Model file for the job. Use its own axes, mm. Face numbers are marked on the shaded views. A direction names the side the tool comes from. Coordinates: 2 decimals unless noted, no trailing zeros. Write each loop counter-clockwise with the first axis right and the second up, starting at its lowest first coordinate (ties: lowest second). Pieces come first, ordered by that corner, then holes. Notation, with made-up numbers: M 74.25,42 L 107.25,42 A32 cw 107.25,81 Z; hole C 25,-1.5 d5. An arc over 180 degrees is marked long. Put each result on its own line as item: value. Start each with the question number.
Q1. Cut at C-C (z = 25.25). Write the cut outline in (x, y).
Q2. Cut at D-D (z = 10.25). Write the cut outline in (x, y).
Q3. Cut at B-B (y = 6.2). Write the cut outline in (x, z).
Q4. Cut at A-A (z = 15). Write the cut outline in (x, y), then the cut area to 3 significant figures.
Q5. Drill centre lines: line 1 along X through (y, z) = (8.5, 21.5); line 2 along Z through (x, y) = (5.15, 6.2); line 3 along X through (y, z) = (2, 1.75). Where is each one in solid material? Low to high.
Q6. Drop flat-ended pins along their axis: pin 1 (3 mm diameter, centred on y = 7.5, z = 16.5, fed in from -X); pin 2 (1.5 mm diameter, centred on x = 2.5, y = 5.5, fed in from +Z); pin 3 (4 mm diameter, centred on x = -29, z = 16.5, fed in from +Y). Give the stop position or say it passes through.
Q7. Pull direction X, two halves, no side cores. Call the marked faces 1, 2 and 3: pulls with the +X half, pulls with the -X half, needs draft (parallel to the pull), parting line crosses it, or undercut.
Q8. Which spindle directions (+Z, -Z, +X, -X, +Y, -Y) get a long thin tool onto all of the face, cutting with end or side? Do the marked faces 4, 5 and 6. Say none if no direction does.
```python
from build123d import *

# Parameters (mm, degrees)
F3_DEPTH = 30
F4_R     = 2.2
F5_DEPTH = 6
F6_W     = 3
F6_H     = 8
F7_DEPTH = 19


with BuildPart() as f3:
    # F2 (on Top) → F3 (new body)
    with BuildSketch(Plane.XY):
        Polygon((0, 13), (0, 0), (6, 0), (6, 19), (-26, 19), (-26, -11), (-34, -11), (-34, -31), (-31, -31), (-31, -14), (-20, -14), (-20, 13), align=None)
    extrude(amount=F3_DEPTH)

    # F4 (on face) → F5 (cut)
    with BuildSketch(Plane(origin=(0, 0, 0), x_dir=(0, -1, 0), z_dir=(-1, 0, 0))):
        with Locations((-6.2, 15)):
            Circle(F4_R)
    extrude(amount=-F5_DEPTH, mode=Mode.SUBTRACT)

    # F6 (on face) → F7 (cut)
    with BuildSketch(Plane.XY.offset(30)):
        with Locations((3, 6.3)):
            Rectangle(F6_W, F6_H)
    extrude(amount=-F7_DEPTH, mode=Mode.SUBTRACT)


solid = f3.part
```
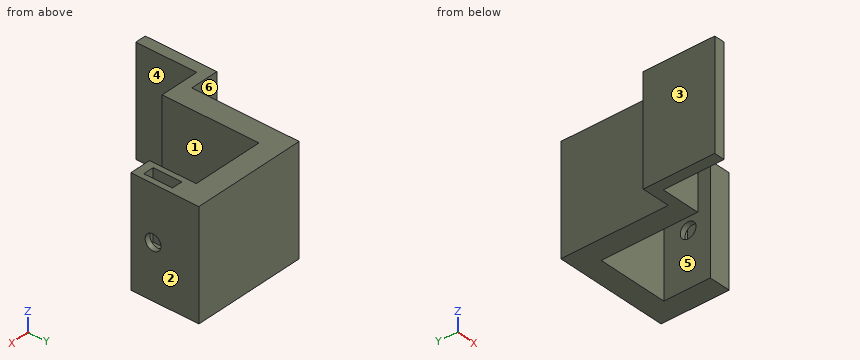
Computed values:
1. outline: M -34,-31 L -31,-31 L -31,-14 L -20,-14 L -20,13 L 0,13 L 0,0 L 6,0 L 6,19 L -26,19 L -26,-11 L -34,-11 Z; hole M 1.5,2.3 L 4.5,2.3 L 4.5,10.3 L 1.5,10.3 Z
2. outline: M -34,-31 L -31,-31 L -31,-14 L -20,-14 L -20,13 L 0,13 L 0,0 L 6,0 L 6,19 L -26,19 L -26,-11 L -34,-11 Z
3. outline: M -26,0 L -20,0 L -20,30 L -26,30 Z; M 0,0 L 6,0 L 6,12.8 L 4.5,12.8 L 4.5,11 L 1.5,11 L 1.5,12.8 L 0,12.8 Z; M 0,17.2 L 1.5,17.2 L 1.5,30 L 0,30 Z; M 4.5,17.2 L 6,17.2 L 6,30 L 4.5,30 Z
4. outline: M -34,-31 L -31,-31 L -31,-14 L -20,-14 L -20,13 L 0,13 L 0,8.4 L 1.5,8.4 L 1.5,10.3 L 4.5,10.3 L 4.5,8.4 L 6,8.4 L 6,19 L -26,19 L -26,-11 L -34,-11 Z; M 0,0 L 6,0 L 6,4 L 4.5,4 L 4.5,2.3 L 1.5,2.3 L 1.5,4 L 0,4 Z
4. area: 470 mm2
5. line 1: -26 to -20, 0 to 1.5, 4.5 to 6
5. line 2: 0 to 12.8, 17.2 to 30
5. line 3: -26 to -20, 0 to 6
6. pin 1: x = -26
6. pin 2: z = 11
6. pin 3: y = -11
7. face 1: undercut
7. face 2: pulls with the +X half
7. face 3: pulls with the -X half
8. face 4: +Z, -Z, +X, -Y
8. face 5: +Z, -Z, -Y
8. face 6: +Z, -Z, -X, +Y
